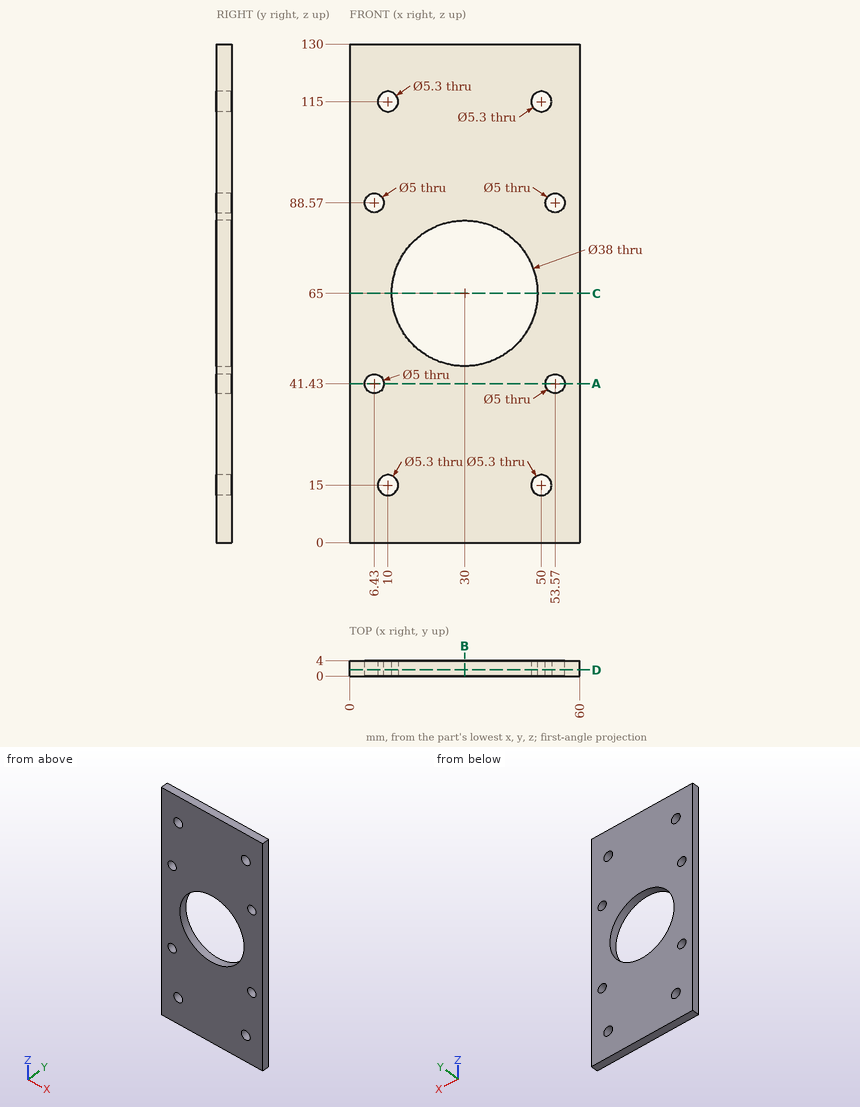
Drawing for the job (mm, zero at the part's lowest x, y, z). Round coordinates to 2 decimals unless told otherwise and drop trailing zeros. Write each loop counter-clockwise with the first axis right and the second up, starting at its lowest first coordinate (ties: lowest second). Pieces come first, ordered by that corner, then holes. Notation, with made-up numbers: (25.5, -24) - (77.5, -24) arc R13 cw to (77.5, -17) - close; hole circle Ø5 at (62, -26.5). An arc over 180 degrees is marked (long way). Write item = value, one per line. Start each with the question number.
Q1. Band-saw the part on B-B (x = 30). Give the cut face in (y, z).
Q2. Probe L1, parallel to X at y = 1.7, z = 115; L2, parallel to X at y = 3, z = 88.57; L3, parallel to Z at x = 10.5, y = 0.85. List the from-to ranges inside material, lowest first. Write a range as from..to.
Q3. Drop a flat-ended pin along its axis: pin 1 (4 mm diameter, centred on x = 10, z = 15, fed in from -Y). Give the stop position or say it passes through.
Q4. Band-saw the part on C-C (z = 65). Give the cut face in (x, y).
Q5. Band-saw the part on A-A (z = 41.43). Give the cut face in (x, y).
Q6. Band-saw the part on D-D (y = 1.6). Count the separate pieces of the cut face and the enclosed holes in it, then the cut area to 3 significant figures.
Answers below:
q1.outline = (0, 0) - (4, 0) - (4, 46) - (0, 46) - close; (0, 84) - (4, 84) - (4, 130) - (0, 130) - close
q2.L1 = 0..7.35, 12.65..47.35, 52.65..60
q2.L2 = 0..3.93, 8.93..51.07, 56.07..60
q2.L3 = 0..12.4, 17.6..112.4, 117.6..130
q3.pin_1 = through
q4.outline = (0, 0) - (11, 0) - (11, 4) - (0, 4) - close; (49, 0) - (60, 0) - (60, 4) - (49, 4) - close
q5.outline = (0, 0) - (3.93, 0) - (3.93, 4) - (0, 4) - close; (8.93, 0) - (51.07, 0) - (51.07, 4) - (8.93, 4) - close; (56.07, 0) - (60, 0) - (60, 4) - (56.07, 4) - close
q6.separate_pieces = 1
q6.enclosed_holes = 9
q6.area = 6,500 mm2
